Part model, mm, in its own coordinate system. Face numbers are marked on the shaded views. A direction names the side the tool comes from. Coordinates: 2 decimals unless noted, no trailing zeros. Order: outer loops, then holes, each group sorted by start corner. A loop starts at its lowest first (then second) coordinate and runs counter-clockwise, first axis right, second up.
1) Tool access for the marked faces 3, 4 and 5: list every direction of +Z, -Z, +X, -X, +Y, -Y with a clear straight run to the whole face (end or side of a thin tool).
2) Cut at D-D (z = -67). List the corners of the cut face in (x, y).
3) Pin check, flat tips, straight feed: pin 1 Ø2.5 at (x, z) = (0, 27.5) entering from +Y; pin 2 Ø1 at (x, z) = (4, -25.5) entering from +Y; pin 3 Ø1 at (x, y) = (-4.5, -3) entering from +Z; pin 4 Ø1.3 at (y, z) = (-3.5, 29) entering from +X. Stop position of each tip, or through.
4) Cut at B-B (y = 0). Give the number of separate pieces and of enclosed holes in the cut face, and give its area (3 significant figures).
5) Cut at A-A (z = 27.5). List the corners of the cut face in (x, y) (3 decimals).
6) Mould opens along Z. For the marked faces 1 and 2 say: +Z half, -Z half, draft (parallel to the pull), parting line (faces both ways), or undercut.
7) Wall check: L1, parallel to Z at x = 4.5, y = -3.5; L2, parallel to Z at x = 0, y = -2.25; L3, parallel to Z at x = 4.75, y = -0.25. Give the ranges that are in metal, low to high.
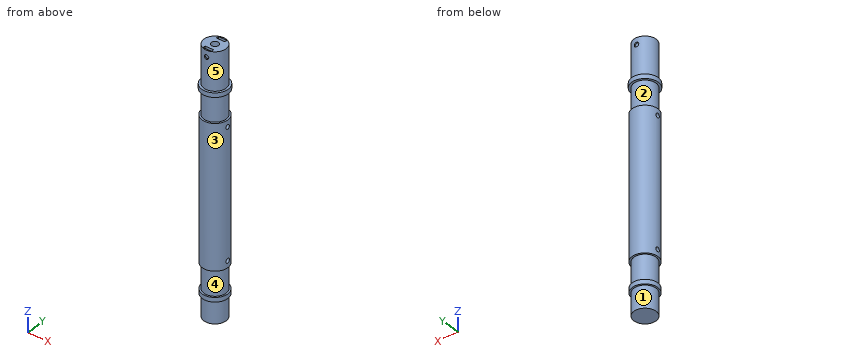
```python
from build123d import *

# Parameters (mm, degrees)
SKETCH1_R           = 6
BOSS_EXTRUDE1_DEPTH = 30.5
SKETCH2_R           = 1.65
CUT_EXTRUDE1_DEPTH  = 14
SKETCH13_W          = 3.9
SKETCH13_H          = 1.2
CUT_EXTRUDE6_DEPTH  = 4.95
SKETCH4_R           = 1
CUT_EXTRUDE7_DEPTH  = 7.5
SKETCH19_R          = 6
SKETCH19_R_2        = 5
CUT_EXTRUDE8_DEPTH  = 45
SKETCH21_R          = 5.8
BOSS_EXTRUDE2_DEPTH = 64
BOSS_EXTRUDE3_START = 13.4
SKETCH22_R          = 5
BOSS_EXTRUDE3_DEPTH = 13.4
BOSS_EXTRUDE5_START = 10
SKETCH24_R          = 5
BOSS_EXTRUDE5_DEPTH = 10
BOSS_EXTRUDE6_START = -19.1
SKETCH25_R          = 6
SKETCH25_R_2        = 5
BOSS_EXTRUDE6_DEPTH = 19.1
CUT_EXTRUDE9_START  = -17.1
SKETCH26_R          = 6
SKETCH26_R_2        = 5
CUT_EXTRUDE9_DEPTH  = 17.1
SKETCH28_R          = 1
CUT_EXTRUDE11_DEPTH = 17
SKETCH23_R          = 5.75
BOSS_EXTRUDE7_DEPTH = 2


with BuildPart() as part:
    # Sketch1 → Boss-Extrude1 (new body)
    with BuildSketch(Plane.XY):
        with Locations(Location((0, 0, 0), (0, 0, 180))):
            Circle(SKETCH1_R)
    extrude(amount=BOSS_EXTRUDE1_DEPTH)

    # Sketch2 → Cut-Extrude1 (cut)
    with BuildSketch(Plane.XY.offset(30.5)):
        Circle(SKETCH2_R)
    extrude(amount=-CUT_EXTRUDE1_DEPTH, mode=Mode.SUBTRACT)

    # Sketch13 → Cut-Extrude6 (cut)
    with BuildSketch(Plane.XY.offset(30.5)):
        with Locations((0, 3.825)):
            Rectangle(SKETCH13_W, SKETCH13_H)
    cut_extrude6 = extrude(amount=-CUT_EXTRUDE6_DEPTH, mode=Mode.SUBTRACT)

    # Sketch4 → Cut-Extrude7 (cut, symmetric)
    with BuildSketch(Plane(origin=(0, 0, 0), x_dir=(1, 0, 0), z_dir=(0, 1, 0))):
        with Locations(Location((0, -27.5, 0), (0, 0, 270))):
            Circle(SKETCH4_R)
    extrude(amount=CUT_EXTRUDE7_DEPTH, both=True, mode=Mode.SUBTRACT)

    # Mirror1: Cut-Extrude6 across plane
    add(cut_extrude6.mirror(Plane.ZX), mode=Mode.SUBTRACT)

    # Sketch19 → Cut-Extrude8 (cut)
    with BuildSketch(Plane(origin=(0, 0, 0), x_dir=(-1, 0, 0), z_dir=(0, 0, -1))):
        Circle(SKETCH19_R)
        Circle(SKETCH19_R_2, mode=Mode.SUBTRACT)
    extrude(amount=-CUT_EXTRUDE8_DEPTH, mode=Mode.SUBTRACT)

    # Sketch21 → Boss-Extrude2 (add)
    with BuildSketch(Plane(origin=(0, 0, 0), x_dir=(-1, 0, 0), z_dir=(0, 0, -1))):
        Circle(SKETCH21_R)
    extrude(amount=BOSS_EXTRUDE2_DEPTH)

    # Sketch22 → Boss-Extrude3 (add)
    with BuildSketch(Plane(origin=(0, 0, -64), x_dir=(-1, 0, 0), z_dir=(0, 0, -1)).offset(BOSS_EXTRUDE3_START)):
        Circle(SKETCH22_R)
    extrude(amount=-BOSS_EXTRUDE3_DEPTH)

    # Sketch24 → Boss-Extrude5 (add)
    with BuildSketch(Plane(origin=(0, 0, -77.4), x_dir=(-1, 0, 0), z_dir=(0, 0, -1)).offset(BOSS_EXTRUDE5_START)):
        Circle(SKETCH24_R)
    extrude(amount=-BOSS_EXTRUDE5_DEPTH)

    # Sketch25 → Boss-Extrude6 (add)
    with BuildSketch(Plane.XY.offset(30.5).offset(BOSS_EXTRUDE6_START)):
        Circle(SKETCH25_R)
        with Locations(Location((0, 0, 0), (0, 0, 180))):
            Circle(SKETCH25_R_2, mode=Mode.SUBTRACT)
    extrude(amount=BOSS_EXTRUDE6_DEPTH)

    # Sketch26 → Cut-Extrude9 (cut)
    with BuildSketch(Plane.XY.offset(30.5).offset(CUT_EXTRUDE9_START)):
        Circle(SKETCH26_R)
        with Locations(Location((0, 0, 0), (0, 0, 180))):
            Circle(SKETCH26_R_2, mode=Mode.SUBTRACT)
    extrude(amount=CUT_EXTRUDE9_DEPTH, mode=Mode.SUBTRACT)

    # Sketch28 → Cut-Extrude11 (cut)
    with BuildSketch(Plane.ZY.offset(5.8)):
        with Locations(Location((-61, 0, 0), (0, 0, 180))):
            Circle(SKETCH28_R)
        with Locations(Location((-3, 0, 0), (0, 0, 180))):
            Circle(SKETCH28_R)
    extrude(amount=-CUT_EXTRUDE11_DEPTH, mode=Mode.SUBTRACT)

    # Sketch23 → Boss-Extrude7 (add)
    with BuildSketch(Plane(origin=(0, 0, -77.4), x_dir=(-1, 0, 0), z_dir=(0, 0, -1))):
        Circle(SKETCH23_R)
    extrude(amount=-BOSS_EXTRUDE7_DEPTH)


solid = part.part
```
Geometry check:
1. face 3: -Z
1. face 4: none
1. face 5: +Z
2. outline: circle Ø10 at (0, 0)
3. pin 1: stops at y = 5
3. pin 2: stops at y = 4.62
3. pin 3: stops at z = 30.5
3. pin 4: stops at x = 4.11
4. separate pieces: 3
4. enclosed holes: 0
4. area: 1,200 mm2
5. outline: (-1.95, -4.425) - (-1.95, -3.225) - (-1, -3.225) - (-1, -1.312) arc R1.65 cw to (-1, 1.312) - (-1, 3.225) - (-1.95, 3.225) - (-1.95, 4.425) - (-1, 4.425) - (-1, 4.899) arc R5 ccw to (-1, -4.899) - (-1, -4.425) - close; (1, -4.899) arc R5 ccw to (1, 4.899) - (1, 4.425) - (1.95, 4.425) - (1.95, 3.225) - (1, 3.225) - (1, 1.312) arc R1.65 cw to (1, -1.312) - (1, -3.225) - (1.95, -3.225) - (1.95, -4.425) - (1, -4.425) - close
6. face 1: draft
6. face 2: undercut
7. L1: z = -77.4 to -75.4, -64 to 0, 11.4 to 13.4
7. L2: z = -87.4 to 26.5, 28.5 to 30.5
7. L3: z = -87.4 to -61.97, -60.03 to -3.97, -2.03 to 30.5
